For this review, take the finished solid that the model builds, in its own axes (mm). A direction names the side the tool comes from. Coordinates: 2 decimals unless noted, no trailing zeros. Loops run counter-clockwise (first coordinate to the right, second up) from the corner with the lowest first, then second, coordinate; pieces in that order, holes last. Notation, with made-up numbers: (60, -25) - (107, -25) arc R7 ccw to (107, -19) - close; hole circle Ø10 at (16, -37.75). An arc over 180 degrees is marked (long way). One line per item, written item: value. Start each with the question number.
1. Take a section at A-A, the plane z = 3.5. State the section outline as (x, y) points.
2. Insertion check: pin 1 (0.8 mm diameter, centred on x = 6, y = 0, fed in from -Z); pin 2 (2 mm diameter, centred on y = -2, z = -2.5, fed in from -X); pin 3 (7 mm diameter, centred on x = 5.81, y = 0, fed in from -Z). Each pin has a flat end and moves straight along its axis. Give the tip position at first contact, or say it passes through.
3. To check wall thickness, follow line 1 (Y direction, x = 6.75, z = -1.25); line 2 (Z direction, x = 0.75, y = 1.5); line 3 (Z direction, x = 9, y = -1.25). State the ranges of each line that lie inside material, in increasing order. Write a range as from..to.
4. For faces 4 (the face through (1.56, 1.34, -3.54)), 5 (the face through (4, -5, -7.9)), 6 (the face through (3.236, 0.811, -2.386)), list the 3-axis set-ups (+Z, -Z, +X, -X, +Y, -Y) from which the entire face can be reached by the end or side of a thin tool; tool diameter is ignored.
5. The part is to be moulded in two halves that separate along X. For faces 1 (the face through (8.033, 0.098, 4.69)), 2 (the face through (6, 0, 4.4)), 3 (the face through (6, 0, 5.9)), say which applies: released by +X, released by -X, zero draft, split by the parting line, or undercut.
6. Take a section at B-B, the plane z = 1.5. State the section outline as (x, y) points.
```python
from build123d import *

# Parameters (mm, degrees)
F2_R = 1


with BuildPart() as f1:
    # F0 (on Front) → F1 (revolve)
    with BuildSketch(Plane.XZ):
        Polygon((5.3116780147, 4.4), (5.8116780147, 4.4), (5.8116780147, 5.9), (4.6192167893, 5.9), (-0.5253184439, -0.1362546736), (1.6116780147, -2.0664450233), (1.6116780147, -3.0388837995), (-0.8728924878, -7.9), (0.8116780147, -7.9), (3.1116780147, -3.4), (3.1116780147, -1.4), (1.5616780147, 0), align=None)
    revolve(axis=Axis((5.8116780147, 0, 1.9449143492), (0, 0, -1)))

    # F2
    f2_edges = [f1.edges().sort_by_distance(p)[0] for p in [
        (12.148674, 0, -0.136255),
        (7.004139, 0, 5.9),
        (10.011678, 0, -2.066445),
        (10.011678, 0, -3.038884),
    ]]
    fillet(f2_edges, radius=F2_R)


solid = f1.part
```
Solutions:
1. outline: circle Ø6.48 at (5.81, 0); hole circle Ø2.53 at (5.81, 0)
2. pin 1: z = 4.3
2. pin 2: x = 1.35
2. pin 3: z = -4.97
3. line 1: -5.02..-2.71, 2.71..5.02
3. line 2: -7.9..-5.15, -1.09..1.1
3. line 3: -4.82..-0.75, 0.97..3.28
4. face 4: none
4. face 5: -Z, +X, -X, +Y, -Y
4. face 6: -Z
5. face 1: split by the parting line
5. face 2: undercut
5. face 3: zero draft
6. outline: circle Ø9.88 at (5.81, 0); hole circle Ø5.94 at (5.81, 0)
